Could you check a few things on this model? Use its own coordinates, in mm. Face numbers are marked on the shaded views. A direction names the side the tool comes from. Coordinates: 2 decimals unless noted, no trailing zeros. Write each loop counter-clockwise with the first axis right and the second up, starting at its lowest first coordinate (ties: lowest second). Pieces come first, ordered by that corner, then holes. Notation, with made-up numbers: (35, -6.75) - (68, -6.75) arc R27 ccw to (68, 10.25) - close; hole circle Ø10 at (82, 24). An arc over 180 degrees is marked (long way). Answer as a JSON object with one key per item and string values. Group by question number.
1) If we section it at B-B (x = 99): Write out the boundary of the cut face in (y, z) (3 decimals), plus the area to 3 significant figures.
2) On a 3-axis mill with a long thin cutter (end or side, diameter ignored), from which of +Z, -Z, +X, -X, +Y, -Y can I reach the whole of each face in a straight line? I mean the marked faces 3, 4, 5 and 6. Say none if no direction works.
3) If we section it at C-C (y = 23): State how many separate pieces and enclosed holes the cut face has, plus the area to 3 significant figures.
4) If we section it at A-A (z = -19): Write out the boundary of the cut face in (x, y) (3 decimals).
5) Please list where these lines run through material, in increasing order: line 1 along Z through (x, y) = (82.5, 20.5); line 2 along Z through (x, y) = (35, 11); line 3 along Z through (x, y) = (146, 27).
6) We'd pull the mould along X, two halves only. Please class the marked faces 1 and 2: released by +X, released by -X, zero draft, split by the parting line, or undercut.
7) Will these pins go through, and if not, where does the flat tip stop? pin 1 Ø11 at (x, z) = (23.96, -154.3) entering from -Y; pin 2 Ø10 at (x, y) = (106.5, 21.5) entering from -Z; pin 3 Ø5 at (y, z) = (16.5, -124.5) entering from +X.
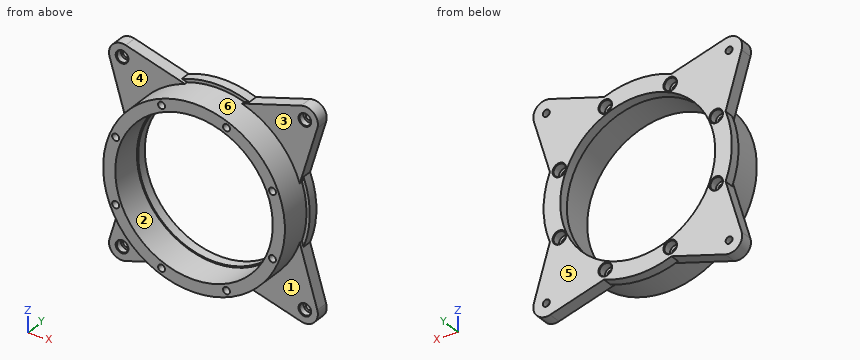
```python
from build123d import *

# Parameters (mm, degrees)
SKETCH2_R                                     = 88.395010725
SKETCH2_R_2                                   = 76.6365
BOSS_EXTRUDE1_DEPTH                           = 40.64
BOSS_EXTRUDE2_START                           = -12.7
BOSS_EXTRUDE2_DEPTH                           = 12.7
CBORE_FOR_1_4_SOCKET_HEAD_CAP_SCREW1_AT_COUNT = 2
CBORE_FOR_1_4_SOCKET_HEAD_CAP_SCREW1_AT_PITCH = 177.8
CBORE_FOR_1_4_SOCKET_HEAD_CAP_SCREW1_2_COUNT  = 2
CBORE_FOR_1_4_SOCKET_HEAD_CAP_SCREW1_2_PITCH  = 251.44717139
CBORE_FOR_1_4_SOCKET_HEAD_CAP_SCREW1_3_COUNT  = 2
CBORE_FOR_1_4_SOCKET_HEAD_CAP_SCREW1_3_PITCH  = 177.8
SKETCH10_R                                    = 91.570010725
SKETCH10_R_2                                  = 75.3865
BOSS_EXTRUDE3_DEPTH                           = 9.525
CBORE_FOR_1_4_BUTTON_HEAD_CAP_SCREW1_AT_COUNT = 2
CBORE_FOR_1_4_BUTTON_HEAD_CAP_SCREW1_AT_PITCH = 63.181034683
CBORE_FOR_1_4_BUTTON_HEAD_CAP_SCREW1_2_COUNT  = 2
CBORE_FOR_1_4_BUTTON_HEAD_CAP_SCREW1_2_PITCH  = 116.743329574
CBORE_FOR_1_4_BUTTON_HEAD_CAP_SCREW1_3_COUNT  = 2
CBORE_FOR_1_4_BUTTON_HEAD_CAP_SCREW1_3_PITCH  = 152.532510818
CBORE_FOR_1_4_BUTTON_HEAD_CAP_SCREW1_4_COUNT  = 2
CBORE_FOR_1_4_BUTTON_HEAD_CAP_SCREW1_4_PITCH  = 165.1
CBORE_FOR_1_4_BUTTON_HEAD_CAP_SCREW1_5_COUNT  = 2
CBORE_FOR_1_4_BUTTON_HEAD_CAP_SCREW1_5_PITCH  = 152.532510818
CBORE_FOR_1_4_BUTTON_HEAD_CAP_SCREW1_6_COUNT  = 2
CBORE_FOR_1_4_BUTTON_HEAD_CAP_SCREW1_6_PITCH  = 116.743329574
CBORE_FOR_1_4_BUTTON_HEAD_CAP_SCREW1_7_COUNT  = 2
CBORE_FOR_1_4_BUTTON_HEAD_CAP_SCREW1_7_PITCH  = 63.181034683


with BuildPart() as part:
    # Sketch2 → Boss-Extrude1 (new body)
    with BuildSketch(Plane(origin=(0, 0, 0), x_dir=(1, 0, 0), z_dir=(0, 1, 0))):
        with Locations(Location((112.864370177, 65.400443246, 0), (0, 0, 270))):
            Circle(SKETCH2_R)
        with Locations(Location((112.864370177, 65.400443246, 0), (0, 0, 270))):
            Circle(SKETCH2_R_2, mode=Mode.SUBTRACT)
    extrude(amount=BOSS_EXTRUDE1_DEPTH)

    # Sketch7 → Boss-Extrude2 (add)
    with BuildSketch(Plane(origin=(0, 40.64, 0), x_dir=(1, 0, 0), z_dir=(0, 1, 0)).offset(BOSS_EXTRUDE2_START)):
        with BuildLine():
            Line((27.586360499, 166.473001979), (85.159974048, 149.341758199))
            ThreePointArc((85.159974048, 149.341758199), (50.359658671, 127.905154752), (28.923055224, 93.104839375))
            Line((28.923055224, 93.104839375), (11.791811444, 150.678452924))
            ThreePointArc((11.791811444, 150.678452924), (14.984114056, 163.280699367), (27.586360499, 166.473001979))
        make_face()
        with BuildLine():
            Line((198.142379855, 166.473001979), (140.568766306, 149.341758199))
            ThreePointArc((140.568766306, 149.341758199), (175.369081684, 127.905154752), (196.805685131, 93.104839375))
            Line((196.805685131, 93.104839375), (213.93692891, 150.678452924))
            ThreePointArc((213.93692891, 150.678452924), (210.744626298, 163.280699367), (198.142379855, 166.473001979))
        make_face()
        with BuildLine():
            Line((213.93692891, -19.877566432), (196.805685131, 37.696047117))
            ThreePointArc((196.805685131, 37.696047117), (175.369081684, 2.89573174), (140.568766306, -18.540871708))
            Line((140.568766306, -18.540871708), (198.142379855, -35.672115487))
            ThreePointArc((198.142379855, -35.672115487), (210.744626298, -32.479812875), (213.93692891, -19.877566432))
        make_face()
        with BuildLine():
            Line((27.586360499, -35.672115487), (85.159974048, -18.540871708))
            ThreePointArc((85.159974048, -18.540871708), (50.359658671, 2.89573174), (28.923055224, 37.696047117))
            Line((28.923055224, 37.696047117), (11.791811444, -19.877566432))
            ThreePointArc((11.791811444, -19.877566432), (14.984114056, -32.479812875), (27.586360499, -35.672115487))
        make_face()
    extrude(amount=BOSS_EXTRUDE2_DEPTH)

    # Sketch9 → CBORE for 1/4 Socket Head Cap Screw1 (revolve, cut)
    with BuildSketch(Plane(origin=(23.964370177, 27.94, 23.499556754), x_dir=(0, 0, -1), z_dir=(1, 0, 0))):
        Polygon((0, 0), (0, 12.7), (3.3782, 12.7), (3.3782, 6.35), (5.55625, 6.35), (5.55625, 0.635), (6.19125, 0), align=None)
    cbore_for_1_4_socket_head_cap_screw1 = revolve(axis=Axis((23.964370177, 21.59, 23.499556754), (0, 1, 0)), mode=Mode.SUBTRACT)

    # CBORE for 1/4 Socket Head Cap Screw1 at: CBORE for 1/4 Socket Head Cap Screw1 ×2
    with Locations(*[(i * CBORE_FOR_1_4_SOCKET_HEAD_CAP_SCREW1_AT_PITCH, 0, 0) for i in range(1, CBORE_FOR_1_4_SOCKET_HEAD_CAP_SCREW1_AT_COUNT)]):
        add(cbore_for_1_4_socket_head_cap_screw1, mode=Mode.SUBTRACT)

    # CBORE for 1_4 Socket Head Cap Screw1 2: CBORE for 1/4 Socket Head Cap Screw1 ×2
    with Locations(*[Vector(0.7071067811865512, 0, -0.7071067811865438) * (i * CBORE_FOR_1_4_SOCKET_HEAD_CAP_SCREW1_2_PITCH) for i in range(1, CBORE_FOR_1_4_SOCKET_HEAD_CAP_SCREW1_2_COUNT)]):
        add(cbore_for_1_4_socket_head_cap_screw1, mode=Mode.SUBTRACT)

    # CBORE for 1_4 Socket Head Cap Screw1 3: CBORE for 1/4 Socket Head Cap Screw1 ×2
    with Locations(*[(0, 0, -i * CBORE_FOR_1_4_SOCKET_HEAD_CAP_SCREW1_3_PITCH) for i in range(1, CBORE_FOR_1_4_SOCKET_HEAD_CAP_SCREW1_3_COUNT)]):
        add(cbore_for_1_4_socket_head_cap_screw1, mode=Mode.SUBTRACT)

    # Sketch10 → Boss-Extrude3 (add)
    with BuildSketch(Plane(origin=(0, 40.64, 0), x_dir=(1, 0, 0), z_dir=(0, 1, 0))):
        with Locations((112.864370177, 65.400443246)):
            Circle(SKETCH10_R)
        with Locations(Location((112.864370177, 65.400443246, 0), (0, 0, 270))):
            Circle(SKETCH10_R_2, mode=Mode.SUBTRACT)
    extrude(amount=-BOSS_EXTRUDE3_DEPTH)

    # Sketch12 → CBORE for 1/4 Button Head Cap Screw1 (revolve, cut)
    with BuildSketch(Plane(origin=(36.598114768, 40.64, -33.809925904), x_dir=(0, 0, 1), z_dir=(1, 0, 0))):
        Polygon((0, 0), (0, 40.64), (3.3782, 40.64), (3.3782, 8.35279), (5.95376, 8.35279), (5.95376, 0.635), (6.58876, 0), align=None)
    cbore_for_1_4_button_head_cap_screw1 = revolve(axis=Axis((36.598114768, 46.99, -33.809925904), (0, -1, 0)), mode=Mode.SUBTRACT)

    # CBORE for 1/4 Button Head Cap Screw1 at: CBORE for 1/4 Button Head Cap Screw1 ×2
    with Locations(*[(0, 0, -i * CBORE_FOR_1_4_BUTTON_HEAD_CAP_SCREW1_AT_PITCH) for i in range(1, CBORE_FOR_1_4_BUTTON_HEAD_CAP_SCREW1_AT_COUNT)]):
        add(cbore_for_1_4_button_head_cap_screw1, mode=Mode.SUBTRACT)

    # CBORE for 1_4 Button Head Cap Screw1 2: CBORE for 1/4 Button Head Cap Screw1 ×2
    with Locations(*[Vector(0.3826834323650937, 0, -0.9238795325112852) * (i * CBORE_FOR_1_4_BUTTON_HEAD_CAP_SCREW1_2_PITCH) for i in range(1, CBORE_FOR_1_4_BUTTON_HEAD_CAP_SCREW1_2_COUNT)]):
        add(cbore_for_1_4_button_head_cap_screw1, mode=Mode.SUBTRACT)

    # CBORE for 1_4 Button Head Cap Screw1 3: CBORE for 1/4 Button Head Cap Screw1 ×2
    with Locations(*[Vector(0.7071067811865462, 0, -0.7071067811865489) * (i * CBORE_FOR_1_4_BUTTON_HEAD_CAP_SCREW1_3_PITCH) for i in range(1, CBORE_FOR_1_4_BUTTON_HEAD_CAP_SCREW1_3_COUNT)]):
        add(cbore_for_1_4_button_head_cap_screw1, mode=Mode.SUBTRACT)

    # CBORE for 1_4 Button Head Cap Screw1 4: CBORE for 1/4 Button Head Cap Screw1 ×2
    with Locations(*[Vector(0.9238795325112864, 0, -0.38268343236509067) * (i * CBORE_FOR_1_4_BUTTON_HEAD_CAP_SCREW1_4_PITCH) for i in range(1, CBORE_FOR_1_4_BUTTON_HEAD_CAP_SCREW1_4_COUNT)]):
        add(cbore_for_1_4_button_head_cap_screw1, mode=Mode.SUBTRACT)

    # CBORE for 1_4 Button Head Cap Screw1 5: CBORE for 1/4 Button Head Cap Screw1 ×2
    with Locations(*[(i * CBORE_FOR_1_4_BUTTON_HEAD_CAP_SCREW1_5_PITCH, 0, 0) for i in range(1, CBORE_FOR_1_4_BUTTON_HEAD_CAP_SCREW1_5_COUNT)]):
        add(cbore_for_1_4_button_head_cap_screw1, mode=Mode.SUBTRACT)

    # CBORE for 1_4 Button Head Cap Screw1 6: CBORE for 1/4 Button Head Cap Screw1 ×2
    with Locations(*[Vector(0.9238795325112864, 0, 0.3826834323650908) * (i * CBORE_FOR_1_4_BUTTON_HEAD_CAP_SCREW1_6_PITCH) for i in range(1, CBORE_FOR_1_4_BUTTON_HEAD_CAP_SCREW1_6_COUNT)]):
        add(cbore_for_1_4_button_head_cap_screw1, mode=Mode.SUBTRACT)

    # CBORE for 1_4 Button Head Cap Screw1 7: CBORE for 1/4 Button Head Cap Screw1 ×2
    with Locations(*[Vector(0.7071067811865459, 0, 0.7071067811865491) * (i * CBORE_FOR_1_4_BUTTON_HEAD_CAP_SCREW1_7_PITCH) for i in range(1, CBORE_FOR_1_4_BUTTON_HEAD_CAP_SCREW1_7_COUNT)]):
        add(cbore_for_1_4_button_head_cap_screw1, mode=Mode.SUBTRACT)


solid = part.part
```
Here are the results:
{
 "1": {"outline": "(0, -152.701) - (31.115, -152.701) - (31.115, -155.915) - (40.64, -155.915) - (40.64, -139.501) - (31.115, -139.501) - (31.115, -140.772) - (0, -140.772) - close; (0, 9.972) - (31.115, 9.972) - (31.115, 8.7) - (40.64, 8.7) - (40.64, 25.114) - (31.115, 25.114) - (31.115, 21.901) - (0, 21.901) - close", "area": "1,060 mm²"},
 "2": {"face 3": "+Z, +X, -Y", "face 4": "+Z, -X, -Y", "face 5": "+Z, -Z, +X, -X, +Y", "face 6": "-Y"},
 "3": {"separate pieces": "1", "enclosed holes": "9", "area": "5,810 mm²"},
 "4": {"outline": "(23.36, 27.94) - (37.627, 27.94) - (37.627, 0) - (51.871, 0) - (51.871, 31.115) - (53.45, 31.115) - (53.45, 40.64) - (23.36, 40.64) - close; (172.279, 31.115) - (173.857, 31.115) - (173.857, 0) - (188.102, 0) - (188.102, 27.94) - (202.369, 27.94) - (202.369, 40.64) - (172.279, 40.64) - close"},
 "5": {"line 1": "z = -148.42 to -144.81, -138.52 to -135.76, 4.96 to 7.72, 14.01 to 17.62", "line 2": "z = -107.24 to -99.97, -94.01 to -36.79, -30.83 to -23.56", "line 3": "z = -147.35 to -144.67, -138.66 to -134.5, 3.7 to 7.86, 13.87 to 16.55"},
 "6": {"face 1": "zero draft", "face 2": "undercut"},
 "7": {"pin 1": "stops at y = 34.29", "pin 2": "stops at z = -153.78", "pin 3": "stops at x = 180.76"}
}
